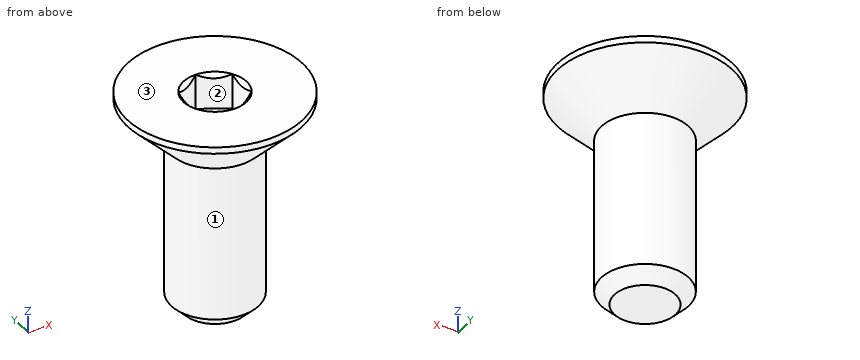
```python
from build123d import *

# Parameters (mm, degrees)
SKETCH3_W          = 10
SKETCH3_H          = 2
CHAMFER1_SIZE      = 0.6
CUT_EXTRUDE1_DEPTH = 1.61
SKETCH9_R          = 1.443375673
CUT_EXTRUDE2_DEPTH = 1.61
CUT_EXTRUDE2_DRAFT = -45


with BuildPart() as part:
    # Sketch3 → Revolve1 (revolve)
    with BuildSketch(Plane(origin=(0, 0, 0), x_dir=(0, 0, -1), z_dir=(1, 0, 0))):
        with Locations((0, 1)):
            Rectangle(SKETCH3_W, SKETCH3_H)
    revolve(axis=Axis((0, 0, -5), (0, 0, 1)))

    # Chamfer1
    chamfer1_edges = [part.edges().sort_by_distance(p)[0] for p in [
        (0, -2, -5),
    ]]
    chamfer(chamfer1_edges, length=CHAMFER1_SIZE)

    # Sketch6 → Revolve2 (revolve)
    with BuildSketch(Plane(origin=(0, 0, 0), x_dir=(0, 0, -1), z_dir=(1, 0, 0))):
        Polygon((-5, 4), (-4.7, 4), (-2.7, 2), (-2.7, 0), (-5, 0), align=None)
    revolve(axis=Axis((0, 0, -5), (0, 0, 1)))

    # Sketch8 → Cut-Extrude1 (cut)
    with BuildSketch(Plane.XY.offset(5)):
        Polygon((0, 1.443375673), (-1.25, 0.721687836), (-1.25, -0.721687836), (0, -1.443375673), (1.25, -0.721687836), (1.25, 0.721687836), align=None)
    extrude(amount=-CUT_EXTRUDE1_DEPTH, mode=Mode.SUBTRACT)


with BuildPart() as cut_extrude2_tool:
    # Sketch9 → Cut-Extrude2 (with draft: the straight prism first)
    with BuildSketch(Plane.XY.offset(5)):
        Circle(SKETCH9_R)
    extrude(amount=-CUT_EXTRUDE2_DEPTH)
    # Cut-Extrude2: the draft: its side faces are tilted about the plane it starts from
    cut_extrude2_sides = [cut_extrude2_tool.faces().sort_by_distance(p)[0] for p in [
        (-1.443375673, 0, 4.195),
    ]]
    draft(cut_extrude2_sides, Plane.XY.offset(5), CUT_EXTRUDE2_DRAFT)


with BuildPart() as part_1:
    add(part.part)

    # Cut-Extrude2: cut by cut_extrude2_tool
    add(cut_extrude2_tool.part, mode=Mode.SUBTRACT)


solid = part_1.part
```
The listing builds one solid part. Answer for the finished solid, in the listing's coordinates (mm). Face numbers are marked on the shaded views. Round coordinates to 2 decimals unless told otherwise and drop trailing zeros. Write each loop counter-clockwise with the first axis right and the second up, starting at its lowest first coordinate (ties: lowest second). Pieces come first, ordered by that corner, then holes. Notation, with made-up numbers: (4, -0.5) -> (22, -0.5) arc R34 ccw to (22, 29.5) -> close; hole circle Ø2 at (72.25, 36.25). An arc over 180 degrees is marked (long way). Answer as a JSON object with one key per item and string values. Group by question number.
Q1. Section C-C (z = 3) is taken. Write down the section's boundary in (x, y), plus the area to 3 significant figures.
Q2. Section A-A (y = 0) is taken. Write down the section's boundary in (x, z).
Q3. Straight lines are drawn through the part: line 1 along X through (y, z) = (-0.5, 3.75); line 2 along X through (y, z) = (-0.25, 4); line 3 along Y through (x, z) = (-1, 3.75). For each, find the intervals that lie inside material, in ascending order.
Q4. Determine the mould class of the marked faces 1, 2 and 3 for opening direction X: pulls with the +X half, pulls with the -X half, needs draft (parallel to the pull), parting line crosses it, or undercut.
Q5. Each of these flat-tipped pins is pushed along its axis until it touches: pin 1 Ø1.5 at (x, z) = (1.5, -3.5) entering from -Y; pin 2 Ø2 at (x, z) = (1, -2) entering from +Y; pin 3 Ø1.5 at (x, z) = (-2.5, -3) entering from -Y. Where does it stop, or does it pass through?
Q6. Section B-B (z = -0.5) is taken. Write down the section's boundary in (x, y).
Check values:
{
 "1": {"outline": "circle Ø4.6 at (0, 0)", "area": "16.6 mm^2"},
 "2": {"outline": "(-4, 4.7) -> (-2, 2.7) -> (-2, -4.4) -> (-1.4, -5) -> (1.4, -5) -> (2, -4.4) -> (2, 2.7) -> (4, 4.7) -> (4, 5) -> (1.44, 5) -> (1.25, 4.81) -> (1.25, 3.39) -> (-1.25, 3.39) -> (-1.25, 4.81) -> (-1.44, 5) -> (-4, 5) -> close"},
 "3": {"line 1": "-3.01 to -1.25, 1.25 to 3.01", "line 2": "-3.29 to -1.25, 1.25 to 3.29", "line 3": "-2.88 to -0.87, 0.87 to 2.88"},
 "4": {"face 1": "parting line crosses it", "face 2": "undercut", "face 3": "needs draft"},
 "5": {"pin 1": "y = -1.85", "pin 2": "y = 2", "pin 3": "y = -0.97"},
 "6": {"outline": "circle Ø4 at (0, 0)"}
}
